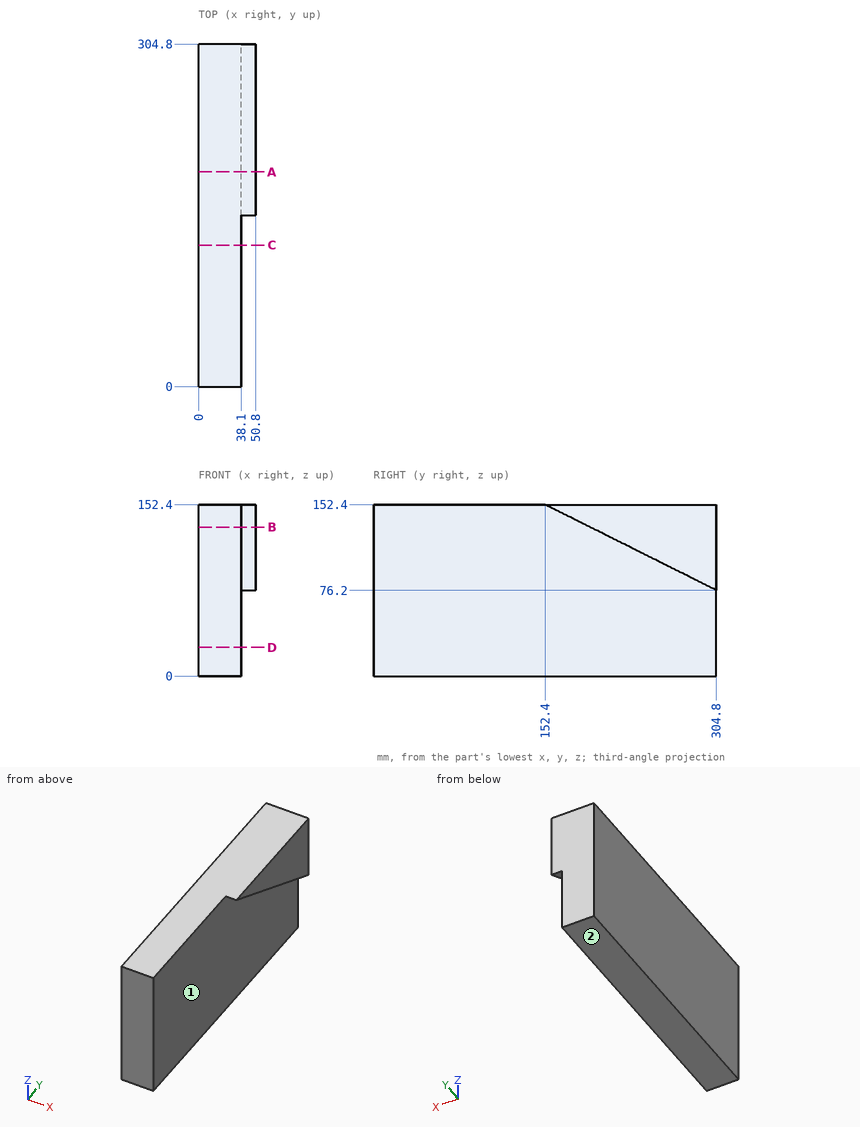
Design review of the part shown in the three views and the two pictorial views. Dimensions are in mm from the part's minimum x, y and z. A direction names the side the tool comes from. Round coordinates to 2 decimals unless told otherwise and drop trailing zeros. Order: outer loops, then holes, each group sorted by start corner. A loop starts at its lowest first (then second) coordinate and runs counter-clockwise, first axis right, second up.
(1) Tool access review of the marked faces 1 and 2: name each direction out of +Z, -Z, +X, -X, +Y, -Y from which nothing blocks a thin tool from reaching the whole face with its end or side.
Working result:
face 1: -Z, +X, -Y
face 2: -Z, +X, -X, +Y, -Y
(2) Wall thickness on L1, parallel to X at y = 92.5, z = 61.5; L2, parallel to Y at x = 47.5, z = 134; L3, parallel to Y at x = 45, z = 81: over which ranges is each line inside the solid? List them lowest first.
Working result:
L1: x = 0 to 38.1
L2: y = 189.2 to 304.8
L3: y = 295.2 to 304.8
(3) Take a section at C-C, the plane y = 126. State the section outline as (x, z) points.
Working result:
outline: (0, 0) - (38.1, 0) - (38.1, 152.4) - (0, 152.4) - close
(4) For P1, Ø8, axis at y = 127.5, z = 46, coming from the +X side; P2, Ø8, axis at x = 44.5, y = 64.5, coming from the +Z side; P3, Ø5, axis at x = 22, z = 24.5, coming from the -Y side, all flat-tipped, find the tip position at first contact; note any pin that passes through.
Working result:
P1: stops at x = 38.1
P2: passes through
P3: stops at y = 0
(5) Take a section at A-A, the plane y = 191. State the section outline as (x, z) points, plus the area to 3 significant figures.
Working result:
outline: (0, 0) - (38.1, 0) - (38.1, 133.1) - (50.8, 133.1) - (50.8, 152.4) - (0, 152.4) - close
area: 6,050 mm2
(6) Take a section at D-D, the plane z = 25.5. State the section outline as (x, y) points, plus the area to 3 significant figures.
Working result:
outline: (0, 0) - (38.1, 0) - (38.1, 304.8) - (0, 304.8) - close
area: 11,600 mm2
(7) Take a section at B-B, the plane z = 132.5. State the section outline as (x, y) points.
Working result:
outline: (0, 0) - (38.1, 0) - (38.1, 192.2) - (50.8, 192.2) - (50.8, 304.8) - (0, 304.8) - close
